from build123d import *

# Parameters (mm, degrees)
F1_DEPTH    = 7
F2_R        = 1.75
F3_DEPTH    = 2.5
F4_R        = 1
F5_DEPTH    = 3
F6_T1_DEPTH = 7.6433659759
F6_T3_DEPTH = 11.4332708022


# Not quite as in the source:
# - a fillet or chamfer that OpenCascade refuses, or shapes differently, is made with other operations: its cross-section is extruded or revolved along the edge and cut away or added


with BuildPart() as f1:
    # F0 (on Top) → F1 (new body)
    with BuildSketch(Plane.XY):
        Polygon((0, 3), (0, 0), (1.53125, 0), (9.46875, 0), (11, 0), (11, 3), align=None)
        Polygon((1.53125, 0), (0, 0), (0, 3), (-2.109375, -10.5), (-2.5, -13), (-0.5, -13), (0.203125, -8.5), (0.515625, -6.5), align=None)
        Polygon((10.484375, -6.5), (0.515625, -6.5), (0.203125, -8.5), (10.796875, -8.5), align=None)
        Polygon((11, 0), (9.46875, 0), (10.484375, -6.5), (10.796875, -8.5), (11.5, -13), (13.5, -13), (13.109375, -10.5), (11, 3), align=None)
        Polygon((19.5, -10.5), (13.109375, -10.5), (13.5, -13), (19.5, -13), align=None)
        Polygon((-2.5, -13), (-2.109375, -10.5), (-8.5, -10.5), (-8.5, -13), align=None)
    extrude(amount=F1_DEPTH)

    # F2 (on face) → F3 (cut, through all)
    with BuildSketch(Plane.XZ.offset(13)):
        with Locations((-5, 3.5)):
            Circle(F2_R)
        with Locations((16, 3.5)):
            Circle(F2_R)
    extrude(amount=-F3_DEPTH, mode=Mode.SUBTRACT)

    # F4 (on face) → F5 (cut, through all)
    with BuildSketch(Plane(origin=(0, 3, 0), x_dir=(-1, 0, 0), z_dir=(0, 1, 0))):
        with Locations((-5.5, 4.75)):
            Circle(F4_R)
    extrude(amount=-F5_DEPTH, mode=Mode.SUBTRACT)

    # F6: chamfer of 1 on 8 edges, made by hand

    # F6_s2 → F6_t1 (cut)
    with BuildSketch(Plane.XZ.offset(7.928317012)):
        Polygon((-7.5, 7), (-8.5, 6), (-8.5, 7), align=None)
        Polygon((-7.5, 0), (-8.5, 1), (-8.5, 0), align=None)
        Polygon((18.5, 7), (19.5, 6), (19.5, 7), align=None)
        Polygon((18.5, 0), (19.5, 1), (19.5, 0), align=None)
    extrude(amount=F6_T1_DEPTH, mode=Mode.SUBTRACT)

    # F6_s4 → F6_t3 (cut)
    with BuildSketch(Plane.XY.offset(-2.2166354011)):
        Polygon((0.8558834213, 3), (-0.1321286125, 2.1543768803), (0, 3), align=None)
        Polygon((10.1441165787, 3), (11.1321286125, 2.1543768803), (11, 3), align=None)
        Polygon((-1.3558834213, -13), (-0.3678713875, -12.1543768803), (-0.5, -13), align=None)
        Polygon((11.3678713875, -12.1543768803), (12.3558834213, -13), (11.5, -13), align=None)
    extrude(amount=F6_T3_DEPTH, mode=Mode.SUBTRACT)


solid = f1.part
The listing builds one solid part. Answer for the finished solid, in the listing's coordinates (mm). A direction names the side the tool comes from. Round coordinates to 2 decimals unless told otherwise and drop trailing zeros. Order: outer loops, then holes, each group sorted by start corner. A loop starts at its lowest first (then second) coordinate and runs counter-clockwise, first axis right, second up. Notation, with made-up numbers: (14, -12.5) -> (68, -12.5) arc R23 cw to (68, 20.5) -> close; hole circle Ø6 at (-35, 67.5). An arc over 180 degrees is marked (long way). One line per item, written item: value.
Item 1: Straight lines are drawn through the part: L1, parallel to Z at x = 5.5, y = 1.35; L2, parallel to Z at x = -5, y = -11.15; L3, parallel to Y at x = 1.75, z = 4.75. For each, find the intervals that lie inside material, in ascending order.
Taken from the geometry:
L1: z = 0 to 3.75, 5.75 to 7
L2: z = 0 to 1.75, 5.25 to 7
L3: y = -8.5 to -6.5, 0 to 3
Item 2: Find section C-C, the plane x = 16. Give the vertices of the cut face in (y, z), then the cut area to 3 significant figures.
Taken from the geometry:
outline: (-13, 0) -> (-10.5, 0) -> (-10.5, 1.75) -> (-13, 1.75) -> close; (-13, 5.25) -> (-10.5, 5.25) -> (-10.5, 7) -> (-13, 7) -> close
area: 8.75 mm2
Item 3: For faces 1 (the flat face through (11.08, -10.3, 3.45)), 2 (the cylindrical face through (6.237, 1.521, 5.426)), 3 (the flat face through (-7, -10.5, 3)), 4 (the flat face through (1.016, -3.295, 3.451)), determine the directions among +Z, -Z, +X, -X, +Y, -Y from which every point of the face is accessible in a straight line to the end or side of a thin tool.
Taken from the geometry:
face 1: +Z, -Z, -Y
face 2: +Y
face 3: +Z, -Z, -X, +Y
face 4: +Z, -Z
Item 4: Find section D-D, the plane y = -3.5. Give the vertices of the cut face in (x, z).
Taken from the geometry:
outline: (-1.02, 0) -> (0.98, 0) -> (0.98, 7) -> (-1.02, 7) -> close; (10.02, 0) -> (12.02, 0) -> (12.02, 7) -> (10.02, 7) -> close
Item 5: Find section A-A, the plane x = 5.5. Give the vertices of the cut face in (y, z), then the cut area to 3 significant figures.
Taken from the geometry:
outline: (-8.5, 0) -> (-6.5, 0) -> (-6.5, 7) -> (-8.5, 7) -> close; (0, 0) -> (3, 0) -> (3, 3.75) -> (0, 3.75) -> close; (0, 5.75) -> (3, 5.75) -> (3, 7) -> (0, 7) -> close
area: 29.0 mm2
Item 6: Find section B-B, the plane z = 2.75. Give the vertices of the cut face in (x, y).
Taken from the geometry:
outline: (-8.5, -13) -> (-6.58, -13) -> (-6.58, -10.5) -> (-8.5, -10.5) -> close; (-3.42, -13) -> (-1.36, -13) -> (-0.37, -12.15) -> (0.2, -8.5) -> (10.8, -8.5) -> (11.37, -12.15) -> (12.36, -13) -> (14.42, -13) -> (14.42, -10.5) -> (13.11, -10.5) -> (11.13, 2.15) -> (10.14, 3) -> (0.86, 3) -> (-0.13, 2.15) -> (-2.11, -10.5) -> (-3.42, -10.5) -> close; (17.58, -13) -> (19.5, -13) -> (19.5, -10.5) -> (17.58, -10.5) -> close; hole (0.52, -6.5) -> (10.48, -6.5) -> (9.47, 0) -> (1.53, 0) -> close
Item 7: For a pull along Y with two mould halves and no side action, classify faces 5 (the flat face through (-0.869, -12.583, 3.451)), 6 (the flat face through (12.135, -4.261, 3.451)), 7 (the flat face through (19, -11.7, 6.5)), 8 (the flat face through (5, 0, 3)) as released by +Y, released by -Y, zero draft, split by the parting line, or undercut.
Taken from the geometry:
face 5: released by -Y
face 6: released by +Y
face 7: zero draft
face 8: undercut
Item 8: Given P1, Ø2, axis at x = -5, z = 3.5, coming from the -Y side; P2, Ø3, axis at x = 17.5, z = 5, coming from the +Y side; P3, Ø5, axis at x = 1, y = 0, coming from the -Z side; P4, Ø1.6, axis at x = 5.5, z = 4.75, coming from the +Y side, each flat-ended and moving along its own axis, determine where each tip first touches the part or whether it passes through.
Taken from the geometry:
P1: passes through
P2: stops at y = -10.5
P3: stops at z = 0
P4: stops at y = -6.5
